CAD build for the part. Positions are in the model's coordinates, mm. Coordinates: 2 decimals unless noted, no trailing zeros. Order: outer loops, then holes, each group sorted by start corner. A loop starts at its lowest first (then second) coordinate and runs counter-clockwise, first axis right, second up. Notation, with made-up numbers: (66, 7) - (113, 7) arc R28 ccw to (113, 35) - close; hole circle Ø10 at (64.25, -28). An arc over 180 degrees is marked (long way). Write each question's results on one line, items separated by ' | '. Start each with the question number.
Q1. Band-saw the part on B-B, the plane z = -13.9. Write the cut outline in (x, y).
Q2. Band-saw the part on A-A, the plane x = -8.5. Write the cut outline in (y, z), then the cut area to 3 significant figures.
Q3. Band-saw the part on D-D, the plane x = 13.5. Write the cut outline in (y, z).
Q4. Band-saw the part on C-C, the plane y = -0.6. Write the cut outline in (x, z).
Q5. Pin check, flat tips, straight feed: P1, Ø1.5, axis at y = -0.5, z = -2, coming from the +X side; P2, Ø5, axis at x = 28.5, z = 0, coming from the -Y side. Stop position of each tip, or through.
Q6. Wall check: probe 1 along X at (y, z) = (-0.75, 0); probe 2 along Z at (x, y) = (15, -1.4); probe 3 along X at (y, z) = (-2, 16). Give the ranges that are in metal, low to high.
Q7. Pull direction Z, two halves, no side cores. Call faces 1 (the cylindrical face through (29.4, -1.48, 2.86)), 2 (the cylindrical face through (-23.122, -1.479, -30.156)), 3 (the flat face through (1, 0, -1)): released by +Z, released by -Z, zero draft, split by the parting line, or undercut.
```python
from build123d import *

# Parameters (mm, degrees)
SKETCH1_R           = 38
SKETCH1_R_2         = 3
SKETCH1_R_3         = 2
BOSS_EXTRUDE1_DEPTH = 3


with BuildPart() as part:
    # Sketch1 → Boss-Extrude1 (new body)
    with BuildSketch(Plane(origin=(0, 0, 0), x_dir=(1, 0, 0), z_dir=(0, 1, 0))):
        with Locations(Location((0, 0, 0), (0, 0, 270))):
            Circle(SKETCH1_R)
        with Locations(Location((28.5, 0, 0), (0, 0, 270))):
            Circle(SKETCH1_R_2, mode=Mode.SUBTRACT)
        with Locations(Location((-28.5, 0, 0), (0, 0, 270))):
            Circle(SKETCH1_R_2, mode=Mode.SUBTRACT)
        with Locations(Location((13.5, 13.9, 0), (0, 0, 270))):
            Circle(SKETCH1_R_2, mode=Mode.SUBTRACT)
        with Locations(Location((13.5, -13.9, 0), (0, 0, 270))):
            Circle(SKETCH1_R_2, mode=Mode.SUBTRACT)
        with Locations(Location((-9.5, 0, 0), (0, 0, 270))):
            Circle(SKETCH1_R_3, mode=Mode.SUBTRACT)
    extrude(amount=-BOSS_EXTRUDE1_DEPTH)


solid = part.part
```
Results below:
1) outline: (-35.37, -3) - (10.5, -3) - (10.5, 0) - (-35.37, 0) - close; (16.5, -3) - (35.37, -3) - (35.37, 0) - (16.5, 0) - close
2) outline: (-3, -37.04) - (0, -37.04) - (0, -1.73) - (-3, -1.73) - close; (-3, 1.73) - (0, 1.73) - (0, 37.04) - (-3, 37.04) - close | area: 212 mm²
3) outline: (-3, -35.52) - (0, -35.52) - (0, -16.9) - (-3, -16.9) - close; (-3, -10.9) - (0, -10.9) - (0, 10.9) - (-3, 10.9) - close; (-3, 16.9) - (0, 16.9) - (0, 35.52) - (-3, 35.52) - close
4) outline: circle Ø76 at (0, 0); hole circle Ø6 at (-28.5, 0); hole circle Ø4 at (-9.5, 0); hole circle Ø6 at (13.5, -13.9); hole circle Ø6 at (13.5, 13.9); hole circle Ø6 at (28.5, 0)
5) P1: stops at x = 37.98 | P2: passes through
6) probe 1: x = -38 to -31.5, -25.5 to -11.5, -7.5 to 25.5, 31.5 to 38 | probe 2: z = -34.91 to -16.5, -11.3 to 11.3, 16.5 to 34.91 | probe 3: x = -34.47 to 11.36, 15.64 to 34.47
7) face 1: undercut | face 2: split by the parting line | face 3: zero draft
